Geometry: see drawing. Coordinates: mm, zero at the bounding-box minimum. Coordinates: 2 decimals unless noted, no trailing zeros. Loops run counter-clockwise (first coordinate to the right, second up) from the corner with the lowest first, then second, coordinate; pieces in that order, holes last. Notation, with made-up numbers: M 40,74.25 L 66,74.25 A22 cw 66,108.25 Z; hole C 65.5,20.25 d3. An arc over 180 degrees is marked long. One line per question, with ' | ' between items. Start each with the question number.
1. Section query B-B, the plane x = 3.2. Output: boundary loops of the cut face in (y, z).
2. Ray query, probe 1 along Y at (x, z) = (1.9, 0.65) (1 decimal); probe 2 along Y at (x, z) = (3.1, 0.7) (1 decimal); probe 3 along X at (y, z) = (37.5, 0.7) (1 decimal). Return the intervals inside material, ascending.
3. Section query C-C, the plane y = 38.5. Output: boundary loops of the cut face in (x, z).
4. Section query A-A, the plane z = 0.5. Output: boundary loops of the cut face in (x, y).
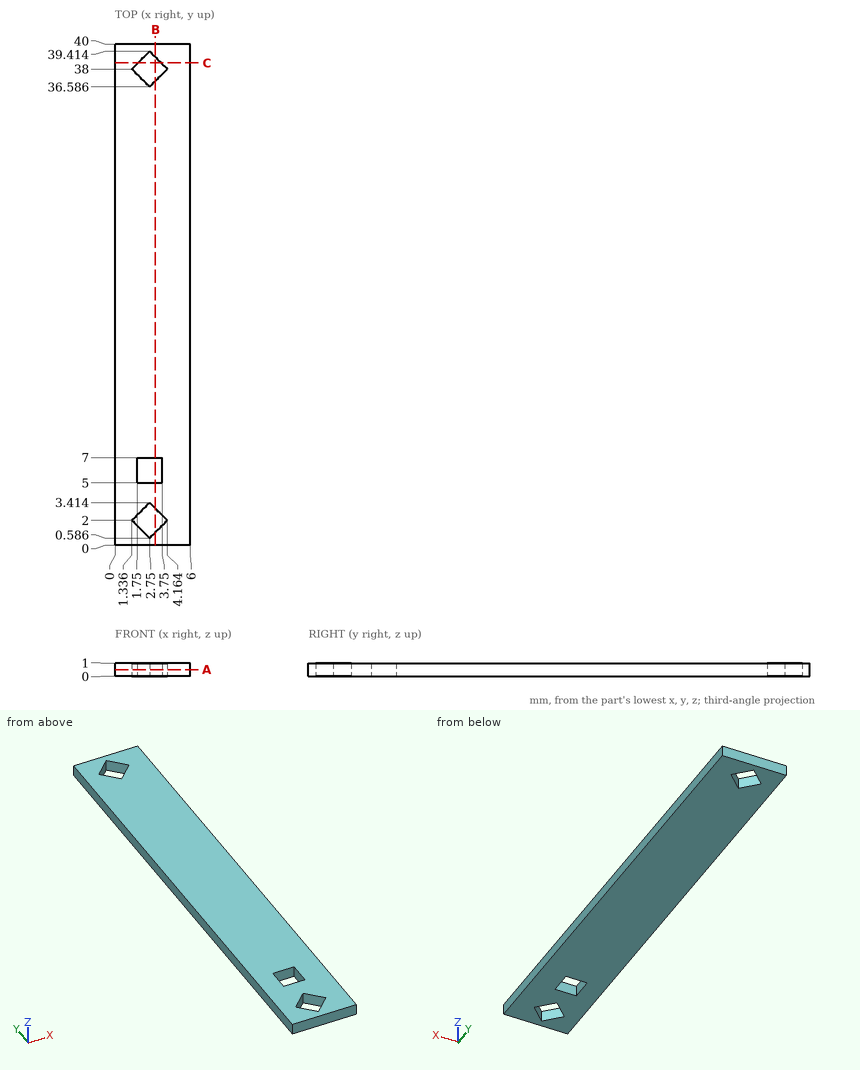
Taken from the geometry:
1) outline: M 0,0 L 1.04,0 L 1.04,1 L 0,1 Z; M 2.96,0 L 5,0 L 5,1 L 2.96,1 Z; M 7,0 L 37.04,0 L 37.04,1 L 7,1 Z; M 38.96,0 L 40,0 L 40,1 L 38.96,1 Z
2) probe 1: 0 to 1.4, 2.6 to 5, 7 to 37.4, 38.6 to 40 | probe 2: 0 to 0.9, 3.1 to 5, 7 to 36.9, 39.1 to 40 | probe 3: 0 to 1.8, 3.7 to 6
3) outline: M 0,0 L 1.84,0 L 1.84,1 L 0,1 Z; M 3.66,0 L 6,0 L 6,1 L 3.66,1 Z
4) outline: M 0,0 L 6,0 L 6,40 L 0,40 Z; hole M 1.34,2 L 2.75,0.59 L 4.16,2 L 2.75,3.41 Z; hole M 1.34,38 L 2.75,36.59 L 4.16,38 L 2.75,39.41 Z; hole M 1.75,5 L 3.75,5 L 3.75,7 L 1.75,7 Z
